Can you work these out from the model? Positions are in its coordinate system, mm. Round coordinates to 2 decimals unless told otherwise and drop trailing zeros. Loops run counter-clockwise (first coordinate to the right, second up) from the corner with the lowest first, then second, coordinate; pieces in that order, holes last. Notation, with made-up numbers: (48, 53.25) -> (102, 53.25) arc R14 cw to (102, 75.25) -> close; hole circle Ø2 at (-2.75, 25). An arc over 180 degrees is marked (long way). Use a Markdown table: item, result.
from build123d import *

# Parameters (mm, degrees)
SKETCH1_W           = 355.6
SKETCH1_H           = 1451.102
BOSS_EXTRUDE1_DEPTH = 0.999998
SKETCH2_W           = 76.45119902
SKETCH2_H           = 12.7
SKETCH2_W_2         = 76.70239804
CUT_EXTRUDE1_DEPTH  = 748.019473372
LPATTERN1_COUNT     = 5
LPATTERN1_PITCH     = 19.05
SKETCH3_W           = 12.7
SKETCH3_H           = 152.4
BOSS_EXTRUDE2_DEPTH = 2.54


with BuildPart() as part:
    # Sketch1 → Boss-Extrude1 (new body)
    with BuildSketch(Plane(origin=(0, 0, 0), x_dir=(0, 0, -1), z_dir=(1, 0, 0))):
        Rectangle(SKETCH1_W, SKETCH1_H)
    extrude(amount=BOSS_EXTRUDE1_DEPTH)

    # Sketch2 → Cut-Extrude1 (cut, through all)
    with BuildSketch(Plane(origin=(0.999998, 0, 0), x_dir=(0, 0, -1), z_dir=(1, 0, 0))):
        with Locations((-88.77440049, 589.382053571)):
            Rectangle(SKETCH2_W, SKETCH2_H)
        with Locations((0.12559951, 589.5101875)):
            Rectangle(SKETCH2_W_2, SKETCH2_H)
        with Locations((88.9, 589.5101875)):
            Rectangle(SKETCH2_W, SKETCH2_H)
    cut_extrude1 = extrude(amount=-CUT_EXTRUDE1_DEPTH, mode=Mode.SUBTRACT)

    # LPattern1: Cut-Extrude1 ×5
    with Locations(*[(0, -i * LPATTERN1_PITCH, 0) for i in range(1, LPATTERN1_COUNT)]):
        add(cut_extrude1, mode=Mode.SUBTRACT)

    # Sketch3 → Boss-Extrude2 (add)
    with BuildSketch(Plane(origin=(0.999998, 0, 0), x_dir=(0, 0, -1), z_dir=(1, 0, 0))):
        with Locations((-158.75, 0)):
            Rectangle(SKETCH3_W, SKETCH3_H)
    extrude(amount=BOSS_EXTRUDE2_DEPTH)


solid = part.part
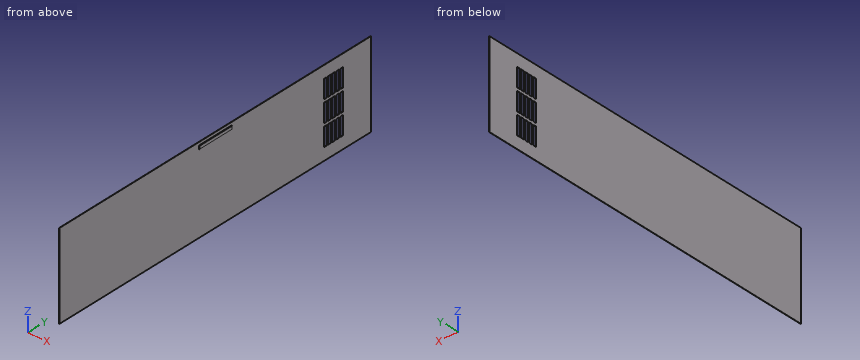
1. I need wall thicknesses on line 1 (Y direction, x = 0.9, z = -67); line 2 (Y direction, x = 0.4, z = 51); line 3 (Z direction, x = 1.6, y = 70.5). Which ranges of each line are inside material? Lowest first, please.
Answer sheet:
| item | result |
|---|---|
| line 1 | y = -725.55 to 506.96, 519.66 to 526.01, 538.71 to 545.06, 557.76 to 564.11, 576.81 to 583.16, 595.86 to 725.55 |
| line 2 | y = -725.55 to 506.83, 519.53 to 525.88, 538.58 to 544.93, 557.63 to 563.98, 576.68 to 583.03, 595.73 to 725.55 |
| line 3 | z = 152.4 to 165.1 |
2. I want a section at B-B (y = 13). Please give me the cut outline in (x, z), plus the area to 3 significant figures.
Answer sheet:
| item | result |
|---|---|
| outline | (0, -177.8) -> (1, -177.8) -> (1, 152.4) -> (3.54, 152.4) -> (3.54, 165.1) -> (1, 165.1) -> (1, 177.8) -> (0, 177.8) -> close |
| area | 388 mm² |
3. I want a section at A-A (z = 22). Please give me the cut outline in (x, y), plus the area to 3 significant figures.
Answer sheet:
| item | result |
|---|---|
| outline | (0, -725.55) -> (1, -725.55) -> (1, 506.96) -> (0, 506.96) -> close; (0, 519.66) -> (1, 519.66) -> (1, 526.01) -> (0, 526.01) -> close; (0, 538.71) -> (1, 538.71) -> (1, 545.06) -> (0, 545.06) -> close; (0, 557.76) -> (1, 557.76) -> (1, 564.11) -> (0, 564.11) -> close; (0, 576.81) -> (1, 576.81) -> (1, 583.16) -> (0, 583.16) -> close; (0, 595.86) -> (1, 595.86) -> (1, 725.55) -> (0, 725.55) -> close |
| area | 1,390 mm² |
4. I want a section at D-D (x = 2.6). Please give me the cut outline in (y, z), plus the area to 3 significant figures.
Answer sheet:
| item | result |
|---|---|
| outline | (-76.2, 152.4) -> (76.2, 152.4) -> (76.2, 165.1) -> (-76.2, 165.1) -> close |
| area | 1,940 mm² |
5. I want a section at C-C (z = -150). Please give me the cut outline in (x, y), plus the area to 3 significant figures.
Answer sheet:
| item | result |
|---|---|
| outline | (0, -725.55) -> (1, -725.55) -> (1, 725.55) -> (0, 725.55) -> close |
| area | 1,450 mm² |
6. Will this pin go through, and if not, where does the flat tip stop? pin 1 Ø1 at (y, z) = (274, 63.5) entering from +X.
Answer sheet:
| item | result |
|---|---|
| pin 1 | stops at x = 1 |
